Check sheet for the modelled part. Datum: model origin and axes. Units: mm. Face numbers are marked on the shaded views. A direction names the side the tool comes from. Give positions to 0.01 mm unless a question says otherwise; leave off trailing zeros. Order: outer loops, then holes, each group sorted by start corner. A loop starts at its lowest first (then second) coordinate and runs counter-clockwise, first axis right, second up. Notation, with made-up numbers: (16, 30) - (73, 30) arc R26 ccw to (73, 44) - close; hole circle Ø8 at (81.5, -28.5). An arc over 180 degrees is marked (long way). Answer in a Markdown table with one row per item.
from build123d import *

# Parameters (mm, degrees)
SKETCH_1_R      = 5
SKETCH_1_R_2    = 2.3
EXTRUDE_1_DEPTH = 5
SKETCH_2_W      = 2
SKETCH_2_H      = 35.417424305
SKETCH_2_W_2    = 35.417424305
SKETCH_2_H_2    = 2
EXTRUDE_2_DEPTH = 5


with BuildPart() as part:
    # ｽｹｯﾁ1 → ﾎﾞｽ - 押し出し1 (new body)
    with BuildSketch(Plane.XY):
        Circle(SKETCH_1_R)
        Circle(SKETCH_1_R_2, mode=Mode.SUBTRACT)
    extrude(amount=EXTRUDE_1_DEPTH)

    # ｽｹｯﾁ2 → ﾎﾞｽ - 押し出し2 (add)
    with BuildSketch(Plane.XY):
        with Locations((1, 22.291287848)):
            Rectangle(SKETCH_2_W, SKETCH_2_H)
        with Locations((-1, 22.291287848)):
            Rectangle(SKETCH_2_W, SKETCH_2_H)
        Polygon((-2, 40), (0, 40), (2, 40), (3.728267906, 42.993447822), (-0.271732094, 42.993447822), align=None)
        Polygon((4.765204655, 45), (3.728267906, 42.993447822), (-0.271732094, 42.993447822), (0.996826512, 45), align=None)
        with Locations((-22.291287848, 1)):
            Rectangle(SKETCH_2_W_2, SKETCH_2_H_2)
        with Locations((-22.291287848, -1)):
            Rectangle(SKETCH_2_W_2, SKETCH_2_H_2)
        Polygon((-40, -2), (-40, 0), (-40, 2), (-45, 4.886751346), (-45, 0.886751346), align=None)
        with Locations((22.291287848, -1)):
            Rectangle(SKETCH_2_W_2, SKETCH_2_H_2)
        with Locations((22.291287848, 1)):
            Rectangle(SKETCH_2_W_2, SKETCH_2_H_2)
        Polygon((45, -4.886751346), (40, -2), (40, 2), (45, -0.886751346), align=None)
        with Locations((1, -22.291287848)):
            Rectangle(SKETCH_2_W, SKETCH_2_H)
        with Locations((-1, -22.291287848)):
            Rectangle(SKETCH_2_W, SKETCH_2_H)
        Polygon((-4.886751346, -45), (-0.886751346, -45), (2, -40), (0, -40), (-2, -40), align=None)
    extrude(amount=EXTRUDE_2_DEPTH)


solid = part.part
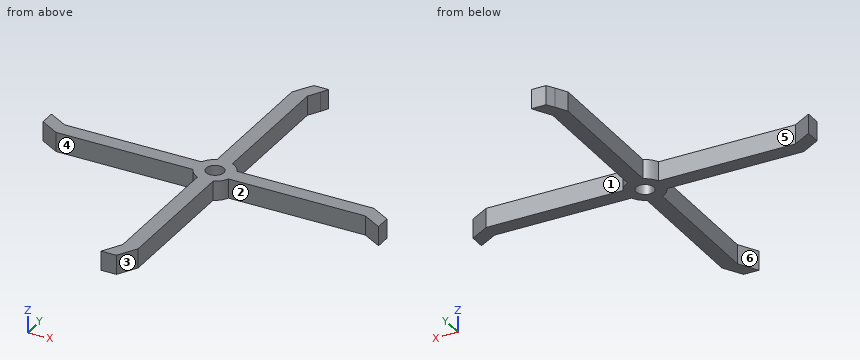
(1) Mould release check, pull along X, two halves, no side actions. Record for the marked faces 4, 5 and 6: pulls with the +X half, pulls with the -X half, needs draft (parallel to the pull), parting line crosses it, or undercut.
Geometry says:
| item | result |
|---|---|
| face 4 | needs draft |
| face 5 | undercut |
| face 6 | pulls with the -X half |
(2) Gauge pin test, flat ends, axial feed: P1, Ø3, axis at x = 21, z = 2.5, coming from the +Y side; P2, Ø2.5, axis at y = 23.5, z = 1.5, coming from the -X side; P3, Ø2.5, axis at x = 19.5, z = 3.5, coming from the -Y side; P4, Ø12, axis at x = -13.5, y = -8.5, coming from the -Z side. Record the tip position at first contact, or that the pin passes through.
Geometry says:
| item | result |
|---|---|
| P1 | y = 2 |
| P2 | x = -2 |
| P3 | y = -2 |
| P4 | through |
(3) Thickness scan on L1, parallel to Y at x = 18, z = 1.05; L2, parallel to Y at x = 0, z = 1.2. Record the ranges inside material, lowest first.
Geometry says:
| item | result |
|---|---|
| L1 | -2 to 2 |
| L2 | -43.46 to -2.3, 2.3 to 43.42 |
(4) Access from +Z, -Z, +X, -X, +Y, -Y to the whole of each face (thin tool, end or side, straight path). Record for the marked faces 1, 2 and 3.
Geometry says:
| item | result |
|---|---|
| face 1 | +Z, -Z, +X, +Y |
| face 2 | +Z, -Z, -Y |
| face 3 | +Z, -Z, +X, -Y |
(5) Cross-section at C-C, the plane y = -30.5. Record the cut outline in (x, z), then the cut area to 3 significant figures.
Geometry says:
| item | result |
|---|---|
| outline | (-2, 0) - (2, 0) - (2, 5) - (-2, 5) - close |
| area | 20.0 mm² |
(6) Cross-section at B-B, the plane x = -3.5. Record the cut outline in (y, z).
Geometry says:
| item | result |
|---|---|
| outline | (-45, 0) - (-42.6, 0) - (-42.6, 5) - (-45, 5) - close; (-3.57, 0) - (3.57, 0) - (3.57, 5) - (-3.57, 5) - close |
(7) Cross-section at A-A, the plane z = 1. Record the cut outline in (x, y).
Geometry says:
| item | result |
|---|---|
| outline | (-45, 0.89) - (-40, -2) - (-4.58, -2) arc R5 ccw to (-2, -4.58) - (-2, -40) - (-4.89, -45) - (-0.89, -45) - (2, -40) - (2, -4.58) arc R5 ccw to (4.58, -2) - (40, -2) - (45, -4.89) - (45, -0.89) - (40, 2) - (4.58, 2) arc R5 ccw to (2, 4.58) - (2, 40) - (3.73, 42.99) - (4.77, 45) - (1, 45) - (-0.27, 42.99) - (-2, 40) - (-2, 4.58) arc R5 ccw to (-4.58, 2) - (-40, 2) - (-45, 4.89) - close; hole circle Ø4.6 at (0, 0) |
